```python
from build123d import *

# Parameters (mm, degrees)
F0_R      = 8
F0_W      = 50
F0_H      = 25
F1_DEPTH  = 30
F3_DEPTH  = 27
F4_R      = 2.55
F5_DEPTH  = 60.001
F4_R_2    = 4.05
F6_DEPTH  = 10
F8_R      = 4.05
F9_DEPTH  = 8
F8_R_2    = 3.025
F10_DEPTH = 50
F8_W      = 90
F8_H      = 31.7965019494
F11_DEPTH = 3
F12_D     = 3.3
F12_DEPTH = 18
F12_TIP   = 0.9914200214
F0_R_2    = 2
F13_DEPTH = 4
F14_DEPTH = 22
F15_DEPTH = 22
F16_DEPTH = 4


with BuildPart() as f1:
    # F0 (on Front) → F1 (new body)
    with BuildSketch(Plane.XZ):
        with BuildLine():
            Line((-20, 39.3), (-20, 0))
            Line((-20, 0), (140, 0))
            Line((140, 0), (140, 39.3))
            Line((140, 39.3), (129.9754699137, 39.3))
            ThreePointArc((129.9754699137, 39.3), (110, 40), (129.9754699137, 40.7))
            Line((129.9754699137, 40.7), (140, 40.7))
            Line((140, 40.7), (140, 60))
            Line((140, 60), (-20, 60))
            Line((-20, 60), (-20, 40.7))
            Line((-20, 40.7), (-9.9754699137, 40.7))
            ThreePointArc((-9.9754699137, 40.7), (0.3502148359, 49.9938655969), (10, 40))
            ThreePointArc((10, 40), (0.3502148359, 30.0061344031), (-9.9754699137, 39.3))
            Line((-9.9754699137, 39.3), (-20, 39.3))
        make_face()
        with Locations((0, 15)):
            Circle(F0_R, mode=Mode.SUBTRACT)
        with Locations((120, 15)):
            Circle(F0_R, mode=Mode.SUBTRACT)
        with Locations((60, 32.5)):
            Rectangle(F0_W, F0_H, mode=Mode.SUBTRACT)
    extrude(amount=F1_DEPTH)

    # F2 (on Top) → F3 (cut)
    with BuildSketch(Plane.XY):
        Polygon((129.1461869532, -12.8157012552), (129.1461869532, -17.2657012552), (133, -19.4907012552), (136.8538130468, -17.2657012552), (136.8538130468, -12.8157012552), (133, -10.5907012552), align=None)
        Polygon((-16.8538130468, -12.8157012552), (-16.8538130468, -17.2657012552), (-13, -19.4907012552), (-9.1461869532, -17.2657012552), (-9.1461869532, -12.8157012552), (-13, -10.5907012552), align=None)
    extrude(amount=F3_DEPTH, mode=Mode.SUBTRACT)

    # F4 (on Top) → F5 (cut, through all)
    with BuildSketch(Plane.XY):
        with Locations((132.991835475, -15.0365363806)):
            Circle(F4_R)
        with Locations((-13.0001418293, -15.0407049805)):
            Circle(F4_R)
    extrude(amount=F5_DEPTH, mode=Mode.SUBTRACT)

    # F4 (on Top) → F6 (cut)
    with BuildSketch(Plane.XY):
        with Locations((-13.0001418293, -15.0407049805)):
            Circle(F4_R_2)
        with Locations((-13.0001418293, -15.0407049805)):
            Circle(F4_R, mode=Mode.SUBTRACT)
        with Locations((132.991835475, -15.0365363806)):
            Circle(F4_R_2)
        with Locations((132.991835475, -15.0365363806)):
            Circle(F4_R, mode=Mode.SUBTRACT)
    extrude(amount=-F6_DEPTH, mode=Mode.SUBTRACT)

    # F8 (on offset) → F9 (cut)
    with BuildSketch(Plane.XY.offset(60)):
        with Locations((-12.9998153025, -15.0684969688)):
            Circle(F8_R)
        with Locations((133.3798532359, -15.0684969688)):
            Circle(F8_R)
    extrude(amount=-F9_DEPTH, mode=Mode.SUBTRACT)

    # F8 (on offset) → F10 (cut)
    with BuildSketch(Plane.XY.offset(60)):
        with Locations((58.9467886905, -15.0684969688)):
            Circle(F8_R_2)
    extrude(amount=-F10_DEPTH, mode=Mode.SUBTRACT)

    # F8 (on offset) → F11 (cut)
    with BuildSketch(Plane.XY.offset(60)):
        with Locations((60, -15.8982509747)):
            Rectangle(F8_W, F8_H)
        with Locations((58.9467886905, -15.0684969688)):
            Circle(F8_R_2, mode=Mode.SUBTRACT)
    extrude(amount=-F11_DEPTH, mode=Mode.SUBTRACT)

    # F12
    with Locations(Plane.XY.offset(60)):
        with Locations((23, -15.0684969688), (97, -15.0684969688)):
            Hole(F12_D / 2, depth=F12_DEPTH)
            with Locations((0, 0, -(F12_DEPTH + F12_TIP / 2))):  # 118° drill point
                Cone(0, F12_D / 2, F12_TIP, mode=Mode.SUBTRACT)

    # F0 (on Front) → F13 (cut)
    with BuildSketch(Plane.XZ):
        Polygon((-0.0046422602, 19.0414518843), (-3.5023211301, 17.0167056269), (-3.4976788699, 12.9752537426), (0.0046422602, 10.9585481157), (3.5023211301, 12.9832943731), (3.4976788699, 17.0247462574), align=None)
        with Locations((0, 15)):
            Circle(F0_R_2, mode=Mode.SUBTRACT)
        Polygon((123.4926623645, 17.0333821434), (119.9853705905, 19.0414254062), (116.492708226, 17.0080432628), (116.5073376355, 12.9666178566), (120.0146294095, 10.9585745938), (123.507291774, 12.9919567372), align=None)
        with Locations((120, 15)):
            Circle(F0_R_2, mode=Mode.SUBTRACT)
    extrude(amount=F13_DEPTH, mode=Mode.SUBTRACT)

    # F0 (on Front) → F14 (join)
    with BuildSketch(Plane.XZ):
        with Locations((120, 15)):
            Circle(F0_R)
        Polygon((116.492708226, 17.0080432628), (119.9853705905, 19.0414254062), (123.4926623645, 17.0333821434), (123.507291774, 12.9919567372), (120.0146294095, 10.9585745938), (116.5073376355, 12.9666178566), align=None, mode=Mode.SUBTRACT)
        with Locations((0, 15)):
            Circle(F0_R)
        Polygon((-3.4976788699, 12.9752537426), (-3.5023211301, 17.0167056269), (-0.0046422602, 19.0414518843), (3.4976788699, 17.0247462574), (3.5023211301, 12.9832943731), (0.0046422602, 10.9585481157), align=None, mode=Mode.SUBTRACT)
    extrude(amount=F14_DEPTH)

    # F0 (on Front) → F15 (join)
    with BuildSketch(Plane.XZ):
        Polygon((123.4926623645, 17.0333821434), (119.9853705905, 19.0414254062), (116.492708226, 17.0080432628), (116.5073376355, 12.9666178566), (120.0146294095, 10.9585745938), (123.507291774, 12.9919567372), align=None)
        with Locations((120, 15)):
            Circle(F0_R_2, mode=Mode.SUBTRACT)
        Polygon((-0.0046422602, 19.0414518843), (-3.5023211301, 17.0167056269), (-3.4976788699, 12.9752537426), (0.0046422602, 10.9585481157), (3.5023211301, 12.9832943731), (3.4976788699, 17.0247462574), align=None)
        with Locations((0, 15)):
            Circle(F0_R_2, mode=Mode.SUBTRACT)
    extrude(amount=F15_DEPTH)

    # F0 (on Front) → F16 (cut)
    with BuildSketch(Plane.XZ):
        Polygon((-0.0046422602, 19.0414518843), (-3.5023211301, 17.0167056269), (-3.4976788699, 12.9752537426), (0.0046422602, 10.9585481157), (3.5023211301, 12.9832943731), (3.4976788699, 17.0247462574), align=None)
        with Locations((0, 15)):
            Circle(F0_R_2, mode=Mode.SUBTRACT)
        Polygon((123.4926623645, 17.0333821434), (119.9853705905, 19.0414254062), (116.492708226, 17.0080432628), (116.5073376355, 12.9666178566), (120.0146294095, 10.9585745938), (123.507291774, 12.9919567372), align=None)
        with Locations((120, 15)):
            Circle(F0_R_2, mode=Mode.SUBTRACT)
    extrude(amount=F16_DEPTH, mode=Mode.SUBTRACT)


solid = f1.part
```
Geometry: final body of the model. Coordinates: model frame, mm. A direction names the side the tool comes from. Coordinates: 2 decimals unless noted, no trailing zeros. Order: outer loops, then holes, each group sorted by start corner. A loop starts at its lowest first (then second) coordinate and runs counter-clockwise, first axis right, second up. Notation, with made-up numbers: M 88.25,36 L 135.25,36 A5 cw 135.25,43 Z; hole C -9,-10.5 d2. An arc over 180 degrees is marked long. Answer in a Markdown table with one row per item. Add a question column.
Q1. Mould query, pull axis Z, two halves, no side actions, for faces 1 (the flat face through (-2, -4, 13)), 2 (the flat face through (-15, -17, 27)), 3 (the cylindrical face through (60.573, -12.518, 51.084)), 4 (the conical face through (23.15, -14.83, 41.18)). Classes: released by +Z, released by -Z, zero draft, split by the parting line, or undercut.
Q2. Section query B-B on z = 37. Return the cut outline in (x, y), and give its area (3 significant figures).
Q3. Section query C-C on x = -6.5. Return the cut outline in (y, z).
Q4. Contact query for flat-ended pins moving along their axis: P1, Ø6.5, axis at x = 0, z = 15, coming from the +Y side; P2, Ø4, axis at x = 83.5, y = -5.5, coming from the +Z side; P3, Ø4.5, axis at x = -13, y = -15.04, coming from the -Z side; P4, Ø2.5, axis at x = -14.5, y = -15.5, coming from the +Z side. Output: stop coordinate, or through.
Q5. Section query A-A on y = -2.5. Count the separate pieces of the cut face and the enclosed holes in it, and give its area (3 significant figures).
Q6. Line query: L1, parallel to Z at x = 0, y = -25; L2, parallel to X at y = -14.75, z = 28; L3, parallel to X at y = -5.5, z = 34. Output: solid intervals per line, ascending.
Q7. Reachability of faces 5 (the flat face through (-14.9, -11.688, 13.311)), 6 (the cylindrical face through (-1.73, -25.94, 7.19)), 7 (the flat face through (135, -17, 52)), 8 (the flat face through (-1.729, -1.972, 18.043)) from +Z, -Z, +X, -X, +Y, -Y: full face, straight path, thin tool, end or side. Return the list, or none.
Completed:
| question | item | result |
|---|---|---|
| 1 | face 1 | undercut |
| 1 | face 2 | released by -Z |
| 1 | face 3 | zero draft |
| 1 | face 4 | released by +Z |
| 2 | outline | M -20,-30 L -9.54,-30 L -9.54,0 L -20,0 Z; M 9.54,-30 L 35,-30 L 35,0 L 9.54,0 Z; M 85,-30 L 110.46,-30 L 110.46,0 L 85,0 Z; M 129.54,-30 L 140,-30 L 140,0 L 129.54,0 Z; hole C -13,-15.04 d5.1; hole C 132.99,-15.04 d5.1 |
| 2 | area | 2,110 mm2 |
| 3 | outline | M -30,0 L 0,0 L 0,32.4 L -30,32.4 L -30,19.66 L -22,19.66 L -22,10.34 L -30,10.34 Z; M -30,47.6 L 0,47.6 L 0,60 L -30,60 Z |
| 4 | P1 | stops at y = -4 |
| 4 | P2 | stops at z = 57 |
| 4 | P3 | passes through |
| 4 | P4 | stops at z = 52 |
| 5 | separate pieces | 1 |
| 5 | enclosed holes | 3 |
| 5 | area | 7,340 mm2 |
| 6 | L1 | z = 0 to 7, 23 to 30, 50 to 60 |
| 6 | L2 | x = -20 to -15.53, -10.47 to 35, 85 to 130.46, 135.53 to 140 |
| 6 | L3 | x = -20 to -8, 8 to 35, 85 to 112, 128 to 140 |
| 7 | face 5 | -Z |
| 7 | face 6 | -Y |
| 7 | face 7 | +Z |
| 7 | face 8 | +Y |
